The listing builds one solid part. Answer for the finished solid, in the listing's coordinates (mm). Face numbers are marked on the shaded views. A direction names the side the tool comes from. Give positions to 0.01 mm unless a question says otherwise; leave off trailing zeros. Order: outer loops, then holes, each group sorted by start corner. A loop starts at its lowest first (then second) coordinate and runs counter-clockwise, first axis right, second up. Notation, with made-up numbers: (-34, 79) - (14, 79) arc R7 ccw to (14, 90) - close; hole circle Ø4 at (66.25, 85). An arc over 180 degrees is marked (long way). Answer as CSV lines item,"result". Start each with the question number.
1. Section B-B on y = -23 is taken. Give the vertices of the cut face in (x, z), and give its area (3 significant figures).
2. Section A-A on x = -25 is taken. Give the vertices of the cut face in (y, z).
3. Consider line 1 along Y through (x, z) = (23, 3.75); line 2 along Y through (x, z) = (-25, 2.25); line 3 along X through (y, z) = (-0.5, 5.5). Determine where each line is inside the solid, lowest interval first. Write a range as [from, to].
4. Which of the six approach directions +Z, -Z, +X, -X, +Y, -Y give full straight-line access (tool end or side, diameter ignored) to the marked faces 4 and 5?
5. Determine the mould class of the marked faces 1, 2 and 3 for opening direction Y: +Y half, -Y half, draft (parallel to the pull), parting line (faces both ways), or undercut.
6. Section D-D on y = -9 is taken. Give the vertices of the cut face in (x, z), and give its area (3 significant figures).
7. Flat-ended cylindrical pins translate along their axes: pin 1 (1.5 mm diameter, centred on x = -7.5, y = -21, fed in from +Z); pin 2 (1 mm diameter, centred on x = -21.5, z = 7.5, fed in from +Y); pin 3 (5 mm diameter, centred on x = 23, y = 25, fed in from +Z); pin 4 (1.5 mm diameter, centred on x = -14.5, z = 4.5, fed in from -Y). Find the tip coordinate at first contact, or state that the pin passes through.
8. Section C-C on z = 6.25 is taken. Count the separate pieces of the cut face and the enclosed holes in it, and give its area (3 significant figures).
from build123d import *

# Parameters (mm, degrees)
SKETCH1_R           = 40
BOSS_EXTRUDE1_DEPTH = 10
SKETCH2_R           = 27.5
CUT_EXTRUDE1_DEPTH  = 6.5
SKETCH3_R           = 4
CUT_EXTRUDE2_DEPTH  = 58.445626465


with BuildPart() as part:
    # Sketch1 → Boss-Extrude1 (new body)
    with BuildSketch(Plane.XY):
        Circle(SKETCH1_R)
    extrude(amount=BOSS_EXTRUDE1_DEPTH)

    # Sketch2 → Cut-Extrude1 (cut)
    with BuildSketch(Plane.XY.offset(10)):
        Circle(SKETCH2_R)
    extrude(amount=-CUT_EXTRUDE1_DEPTH, mode=Mode.SUBTRACT)

    # Sketch3 → Cut-Extrude2 (cut, through all)
    with BuildSketch(Plane.XY.offset(10)):
        with Locations((-25, 23)):
            Circle(SKETCH3_R)
        with Locations((-1.414213562, 33.941125497)):
            Circle(SKETCH3_R)
        with Locations((23, 25)):
            Circle(SKETCH3_R)
        with Locations((33.941125497, 1.414213562)):
            Circle(SKETCH3_R)
        with Locations((25, -23)):
            Circle(SKETCH3_R)
        with Locations((1.414213562, -33.941125497)):
            Circle(SKETCH3_R)
        with Locations((-23, -25)):
            Circle(SKETCH3_R)
        with Locations((-33.941125497, -1.414213562)):
            Circle(SKETCH3_R)
    extrude(amount=-CUT_EXTRUDE2_DEPTH, mode=Mode.SUBTRACT)


solid = part.part
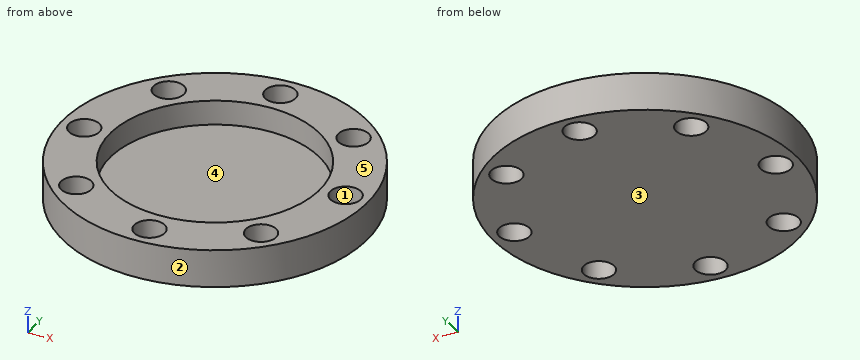
Checks:
1,outline,"(-32.73, 0) - (-26.46, 0) - (-26.46, 10) - (-32.73, 10) - close; (-19.54, 0) - (21, 0) - (21, 10) - (15.07, 10) - (15.07, 3.5) - (-15.07, 3.5) - (-15.07, 10) - (-19.54, 10) - close; (29, 0) - (32.73, 0) - (32.73, 10) - (29, 10) - close"
1,area,"309 mm²"
2,outline,"(-31.22, 0) - (-28.46, 0) - (-28.46, 10) - (-31.22, 10) - close; (-21.54, 0) - (19, 0) - (19, 10) - (11.46, 10) - (11.46, 3.5) - (-11.46, 3.5) - (-11.46, 10) - (-21.54, 10) - close; (27, 0) - (31.22, 0) - (31.22, 10) - (27, 10) - close"
3,line 1,"y = [-32.73, -26.46], [-19.54, -15.07], [15.07, 21], [29, 32.73]"
3,line 2,"y = [-31.22, -28.46], [-21.54, 19], [27, 31.22]"
3,line 3,"x = [-40, -37.84], [-30.05, -27.5], [27.5, 30.43], [37.45, 40]"
4,face 4,"+Z"
4,face 5,"+Z, +X, -X, +Y, -Y"
5,face 1,"undercut"
5,face 2,"parting line"
5,face 3,"draft"
6,outline,"(-38.97, 0) - (38.97, 0) - (38.97, 10) - (25.99, 10) - (25.99, 3.5) - (-25.99, 3.5) - (-25.99, 10) - (-38.97, 10) - close"
6,area,"442 mm²"
7,pin 1,"stops at z = 3.5"
7,pin 2,"stops at y = 34.04"
7,pin 3,"passes through"
7,pin 4,"stops at y = -37.56"
8,separate pieces,"1"
8,enclosed holes,"9"
8,area,"2,250 mm²"
